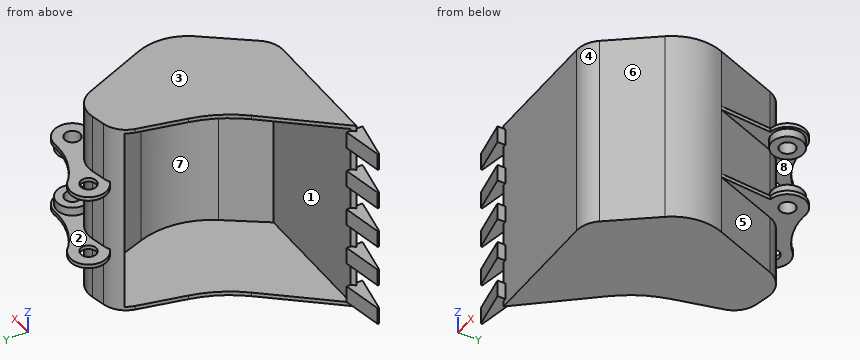
from build123d import *

# Parameters (mm, degrees)
BOSS_EXTRUDE4_DEPTH = 375
BOSS_EXTRUDE5_DEPTH = 7.5
CUT_EXTRUDE1_DEPTH  = 360
BOSS_EXTRUDE6_DEPTH = 32.5
LPATTERN1_COUNT     = 3
LPATTERN1_PITCH     = 160
LPATTERN1_COL_COUNT = 3
LPATTERN1_COL_PITCH = 160
SKETCH11_R          = 30
CUT_EXTRUDE2_DEPTH  = 1263.512529339
SKETCH12_R          = 60
SKETCH12_R_2        = 30
BOSS_EXTRUDE7_DEPTH = 32.5


with BuildPart() as part:
    # Sketch1 → Boss-Extrude4 (new, symmetric)
    with BuildSketch(Plane.XY):
        with BuildLine():
            Line((281.569977344, 264.00526259), (60.043258876, 0))
            Line((60.043258876, 0), (520.65961219, 0))
            ThreePointArc((520.65961219, 0), (564.907123778, 10.321921752), (600.02024832, 39.156845634))
            Line((600.02024832, 39.156845634), (730.44724808, 209.279019234))
            ThreePointArc((730.44724808, 209.279019234), (769.910899903, 304.081580706), (757.128519442, 405.97130652))
            Line((757.128519442, 405.97130652), (658.940406775, 648.676304078))
            ThreePointArc((658.940406775, 648.676304078), (613.16613298, 699.478789474), (545.447965883, 708.988074874))
            Line((545.447965883, 708.988074874), (493.401915404, 697.925345336))
            ThreePointArc((493.401915404, 697.925345336), (444.503904969, 671.828213907), (417.014937982, 623.698884104))
            Line((417.014937982, 623.698884104), (374.151637205, 447.112342165))
            ThreePointArc((374.151637205, 447.112342165), (338.436231819, 350.211710608), (281.569977344, 264.00526259))
        make_face()
    extrude(amount=BOSS_EXTRUDE4_DEPTH, both=True)

    # Sketch6 → Boss-Extrude5 (add, symmetric)
    with BuildSketch(Plane.XY.offset(140)):
        with BuildLine():
            Line((739.837232288, 602.21499348), (757.128519442, 405.97130652))
            Line((757.128519442, 405.97130652), (468.079651675, 688.843619215))
            ThreePointArc((468.079651675, 688.843619215), (438.909700759, 795.263431413), (549.226629435, 797.76097261))
            ThreePointArc((549.226629435, 797.76097261), (629.357941615, 754.030269249), (719.665800913, 740.692647386))
            ThreePointArc((719.665800913, 740.692647386), (801.063667795, 681.841548153), (739.837232288, 602.21499348))
        make_face()
    boss_extrude5 = extrude(amount=BOSS_EXTRUDE5_DEPTH, both=True)

    # Mirror2: Boss-Extrude5 across plane
    add(boss_extrude5.mirror(Plane.XY))

    # Sketch7 → Cut-Extrude1 (cut, symmetric)
    with BuildSketch(Plane.XY):
        with BuildLine():
            Line((60.410578327, 15), (329.990480538, 400))
            Line((329.990480538, 400), (404.359842809, 650))
            Line((404.359842809, 650), (608.375948196, 693.364961886))
            Line((608.375948196, 693.364961886), (698.639094975, 432.530508414))
            ThreePointArc((698.639094975, 432.530508414), (712.247197771, 292.899677108), (660.880251772, 162.349355884))
            Line((660.880251772, 162.349355884), (557.705122032, 15))
            Line((557.705122032, 15), (60.410578327, 15))
        make_face()
    extrude(amount=CUT_EXTRUDE1_DEPTH, both=True, mode=Mode.SUBTRACT)

    # Sketch10 → Boss-Extrude6 (add, symmetric)
    with BuildSketch(Plane.XY):
        Polygon((72.542939803, 30), (-77.392739815, 2.5), (-77.392739815, -2.5), (72.542939803, -30), (72.542939803, 0), align=None)
    boss_extrude6 = extrude(amount=BOSS_EXTRUDE6_DEPTH, both=True)

    # LPattern1: Boss-Extrude6 ×3
    with Locations(*[(0, 0, i * LPATTERN1_PITCH) for i in range(1, LPATTERN1_COUNT)]):
        add(boss_extrude6)

    # LPattern1 col: Boss-Extrude6 ×3
    with Locations(*[(0, 0, -i * LPATTERN1_COL_PITCH) for i in range(1, LPATTERN1_COL_COUNT)]):
        add(boss_extrude6)

    # Sketch11 → Cut-Extrude2 (cut, through all)
    with BuildSketch(Plane.XY.offset(147.5)):
        with Locations((495.043258876, 753.442101292)):
            Circle(SKETCH11_R)
        with Locations((731.794701004, 671.751442127)):
            Circle(SKETCH11_R)
    extrude(amount=-CUT_EXTRUDE2_DEPTH, mode=Mode.SUBTRACT)

    # Sketch12 → Boss-Extrude7 (add)
    with BuildSketch(Plane(origin=(0, 0, 132.5), x_dir=(-1, 0, 0), z_dir=(0, 0, -1))):
        with Locations((-731.794701004, 671.751442127)):
            Circle(SKETCH12_R)
        with Locations(Location((-731.794701004, 671.751442127, 0), (0, 0, 180))):
            Circle(SKETCH12_R_2, mode=Mode.SUBTRACT)
    boss_extrude7 = extrude(amount=BOSS_EXTRUDE7_DEPTH)

    # Mirror3: Boss-Extrude7 across plane
    add(boss_extrude7.mirror(Plane.XY))


solid = part.part
The model under review builds one solid part; all positions refer to its coordinate system, in mm. Face numbers are marked on the shaded views. A direction names the side the tool comes from. Give positions to 0.01 mm unless a question says otherwise; leave off trailing zeros. Write each loop counter-clockwise with the first axis right and the second up, starting at its lowest first coordinate (ties: lowest second). Pieces come first, ordered by that corner, then holes. Notation, with made-up numbers: M -2,-26.75 L 45,-26.75 A14 ccw 45,-7.75 Z; hole C 36.5,78 d7. An arc over 180 degrees is marked long. One line per question, with ' | ' between items. Start each with the question number.
Item 1: For the marked faces 5, 6, 7 and 8, list the 3-axis set-ups (+Z, -Z, +X, -X, +Y, -Y) from which the entire face can be reached by the end or side of a thin tool; tool diameter is ignored.
Item 2: Draft analysis for pull direction X (two halves, no side actions). For the marked faces 1, 2, 3 and 4, state which applies: released by +X, released by -X, zero draft, split by the parting line, or undercut.
Item 3: For pin 1 (9 mm diameter, centred on y = -12.5, z = -327, fed in from +X); pin 2 (12 mm diameter, centred on y = 19.5, z = -320.5, fed in from +X); pin 3 (5 mm diameter, centred on y = 190, z = -113.5, fed in from -X), all flat-tipped, find the tip position at first contact; note any pin that passes through.
Item 4: We need section D-D on x = 622.5. Write out the cut boundary in (y, z), plus the area to 3 significant figures.
Item 5: We need section B-B on z = -161.5. Write out the cut boundary in (x, y).
Item 6: We need section A-A on x = 36. Write out the cut boundary in (y, z).
Item 7: We need section C-C on y = 81. Write out the cut boundary in (x, z).
Item 8: Wall thickness on line 1 (Z direction, x = 528.5, y = 331); line 2 (Z direction, x = 699.5, y = 645.5); line 3 (Y direction, x = 149, z = -234): over which ranges is each line inside the solid? List them lowest first. Write a range as from..to.
Results found:
1) face 5: -Z, +X, +Y | face 6: +Z, -Z, +X, -Y | face 7: -X | face 8: none
2) face 1: undercut | face 2: undercut | face 3: zero draft | face 4: released by +X
3) pin 1: stops at x = 72.54 | pin 2: stops at x = 587.37 | pin 3: stops at x = 676.7
4) outline: M 68.48,-375 L 693.85,-375 L 693.85,-147.5 L 756.43,-147.5 L 756.43,-132.5 L 693.85,-132.5 L 693.85,132.5 L 756.43,132.5 L 756.43,147.5 L 693.85,147.5 L 693.85,375 L 68.48,375 Z; hole M 107.54,-360 L 652.55,-360 L 652.55,360 L 107.54,360 Z | area: 78,500 mm2
5) outline: M -77.39,-2.5 L 72.54,-30 L 72.54,0 L 520.66,0 A100 ccw 600.02,39.16 L 730.45,209.28 A200 ccw 757.13,405.97 L 658.94,648.68 A100 ccw 545.45,708.99 L 493.4,697.93 A100 ccw 431.05,655.67 L 608.38,693.36 L 698.64,432.53 A300 cw 660.88,162.35 L 557.71,15 L 72.63,15 L 72.54,14.9 L 72.54,30 L -77.39,2.5 Z
6) outline: M -23.3,-352.5 L 23.3,-352.5 L 23.3,-287.5 L -23.3,-287.5 Z; M -23.3,-192.5 L 23.3,-192.5 L 23.3,-127.5 L -23.3,-127.5 Z; M -23.3,-32.5 L 23.3,-32.5 L 23.3,32.5 L -23.3,32.5 Z; M -23.3,127.5 L 23.3,127.5 L 23.3,192.5 L -23.3,192.5 Z; M -23.3,287.5 L 23.3,287.5 L 23.3,352.5 L -23.3,352.5 Z
7) outline: M 128.01,-375 L 632.1,-375 L 632.1,375 L 128.01,375 L 128.01,360 L 603.92,360 L 603.92,-360 L 128.01,-360 Z
8) line 1: z = -375..-360, 360..375 | line 2: z = -147.5..-100, 100..147.5 | line 3: y = 0..15
